from build123d import *

# Parameters (mm, degrees)
SKETCH_1_R             = 87
SM_BASE_FLANGE_1_DEPTH = 3
CUT_EXTRUDE_1_REACH    = 125.073
SKETCH_6_R             = 6.1
SKETCH_6_R_2           = 1
SKETCH_6_R_3           = 4.1
SKETCH_6_R_4           = 1.5
SKETCH_6_W             = 10
SKETCH_6_H             = 20
SKETCH_6_W_2           = 20
SKETCH_6_H_2           = 10
FILLET_1_R             = 3


# Sheet-metal steps are written as plain solids
with BuildPart() as part:
    # Sketch 1 → 基体-法兰1 (new body)
    with BuildSketch(Plane(origin=(0, 0, 0), x_dir=(1, 0, 0), z_dir=(0, 1, 0))):
        with Locations(Location((0, 0, 0), (0, 0, 270))):
            Circle(SKETCH_1_R)
    extrude(amount=-SM_BASE_FLANGE_1_DEPTH)

    # 草图6 → 切除-拉伸1 (cut, up to next)
    with BuildSketch(Plane(origin=(0, 0, 0), x_dir=(1, 0, 0), z_dir=(0, 1, 0)), mode=Mode.PRIVATE) as cut_extrude_1_sk1:
        with Locations(Location((0, 0, 0), (0, 0, 270))):
            Circle(SKETCH_6_R)
    cut_extrude_1_tool1 = extrude(cut_extrude_1_sk1.sketch, amount=-CUT_EXTRUDE_1_REACH, mode=Mode.PRIVATE) & part.part
    # 草图6 → 切除-拉伸1 (cut, up to next)
    with BuildSketch(Plane(origin=(0, 0, 0), x_dir=(1, 0, 0), z_dir=(0, 1, 0)), mode=Mode.PRIVATE) as cut_extrude_1_sk2:
        with Locations(Location((-8, 9.15, 0), (0, 0, 270))):
            Circle(SKETCH_6_R_2)
    cut_extrude_1_tool2 = extrude(cut_extrude_1_sk2.sketch, amount=-CUT_EXTRUDE_1_REACH, mode=Mode.PRIVATE) & part.part
    # 草图6 → 切除-拉伸1 (cut, up to next)
    with BuildSketch(Plane(origin=(0, 0, 0), x_dir=(1, 0, 0), z_dir=(0, 1, 0)), mode=Mode.PRIVATE) as cut_extrude_1_sk3:
        with Locations(Location((-7, 20.15, 0), (0, 0, 270))):
            Circle(SKETCH_6_R_2)
    cut_extrude_1_tool3 = extrude(cut_extrude_1_sk3.sketch, amount=-CUT_EXTRUDE_1_REACH, mode=Mode.PRIVATE) & part.part
    # 草图6 → 切除-拉伸1 (cut, up to next)
    with BuildSketch(Plane(origin=(0, 0, 0), x_dir=(1, 0, 0), z_dir=(0, 1, 0)), mode=Mode.PRIVATE) as cut_extrude_1_sk4:
        with Locations(Location((53.033008589, 53.033008589, 0), (0, 0, 270))):
            Circle(SKETCH_6_R_3)
    cut_extrude_1_tool4 = extrude(cut_extrude_1_sk4.sketch, amount=-CUT_EXTRUDE_1_REACH, mode=Mode.PRIVATE) & part.part
    # 草图6 → 切除-拉伸1 (cut, up to next)
    with BuildSketch(Plane(origin=(0, 0, 0), x_dir=(1, 0, 0), z_dir=(0, 1, 0)), mode=Mode.PRIVATE) as cut_extrude_1_sk5:
        with Locations(Location((-53.033008589, 53.033008589, 0), (0, 0, 270))):
            Circle(SKETCH_6_R_3)
    cut_extrude_1_tool5 = extrude(cut_extrude_1_sk5.sketch, amount=-CUT_EXTRUDE_1_REACH, mode=Mode.PRIVATE) & part.part
    # 草图6 → 切除-拉伸1 (cut, up to next)
    with BuildSketch(Plane(origin=(0, 0, 0), x_dir=(1, 0, 0), z_dir=(0, 1, 0)), mode=Mode.PRIVATE) as cut_extrude_1_sk6:
        with Locations(Location((53.033008589, -53.033008589, 0), (0, 0, 270))):
            Circle(SKETCH_6_R_3)
    cut_extrude_1_tool6 = extrude(cut_extrude_1_sk6.sketch, amount=-CUT_EXTRUDE_1_REACH, mode=Mode.PRIVATE) & part.part
    # 草图6 → 切除-拉伸1 (cut, up to next)
    with BuildSketch(Plane(origin=(0, 0, 0), x_dir=(1, 0, 0), z_dir=(0, 1, 0)), mode=Mode.PRIVATE) as cut_extrude_1_sk7:
        with Locations(Location((-53.033008589, -53.033008589, 0), (0, 0, 270))):
            Circle(SKETCH_6_R_3)
    cut_extrude_1_tool7 = extrude(cut_extrude_1_sk7.sketch, amount=-CUT_EXTRUDE_1_REACH, mode=Mode.PRIVATE) & part.part
    # 草图6 → 切除-拉伸1 (cut, up to next)
    with BuildSketch(Plane(origin=(0, 0, 0), x_dir=(1, 0, 0), z_dir=(0, 1, 0)), mode=Mode.PRIVATE) as cut_extrude_1_sk8:
        with Locations(Location((8, 9.15, 0), (0, 0, 270))):
            Circle(SKETCH_6_R_2)
    cut_extrude_1_tool8 = extrude(cut_extrude_1_sk8.sketch, amount=-CUT_EXTRUDE_1_REACH, mode=Mode.PRIVATE) & part.part
    # 草图6 → 切除-拉伸1 (cut, up to next)
    with BuildSketch(Plane(origin=(0, 0, 0), x_dir=(1, 0, 0), z_dir=(0, 1, 0)), mode=Mode.PRIVATE) as cut_extrude_1_sk9:
        with Locations(Location((7, 20.15, 0), (0, 0, 270))):
            Circle(SKETCH_6_R_2)
    cut_extrude_1_tool9 = extrude(cut_extrude_1_sk9.sketch, amount=-CUT_EXTRUDE_1_REACH, mode=Mode.PRIVATE) & part.part
    # 草图6 → 切除-拉伸1 (cut, up to next)
    with BuildSketch(Plane(origin=(0, 0, 0), x_dir=(1, 0, 0), z_dir=(0, 1, 0)), mode=Mode.PRIVATE) as cut_extrude_1_sk10:
        with Locations(Location((0, 27.15, 0), (0, 0, 270))):
            Circle(SKETCH_6_R_2)
    cut_extrude_1_tool10 = extrude(cut_extrude_1_sk10.sketch, amount=-CUT_EXTRUDE_1_REACH, mode=Mode.PRIVATE) & part.part
    # 草图6 → 切除-拉伸1 (cut, up to next)
    with BuildSketch(Plane(origin=(0, 0, 0), x_dir=(1, 0, 0), z_dir=(0, 1, 0)), mode=Mode.PRIVATE) as cut_extrude_1_sk11:
        with Locations(Location((-36.769552622, -36.769552622, 0), (0, 0, 270))):
            Circle(SKETCH_6_R_4)
    cut_extrude_1_tool11 = extrude(cut_extrude_1_sk11.sketch, amount=-CUT_EXTRUDE_1_REACH, mode=Mode.PRIVATE) & part.part
    # 草图6 → 切除-拉伸1 (cut, up to next)
    with BuildSketch(Plane(origin=(0, 0, 0), x_dir=(1, 0, 0), z_dir=(0, 1, 0)), mode=Mode.PRIVATE) as cut_extrude_1_sk12:
        with Locations(Location((-36.769552622, 36.769552622, 0), (0, 0, 270))):
            Circle(SKETCH_6_R_4)
    cut_extrude_1_tool12 = extrude(cut_extrude_1_sk12.sketch, amount=-CUT_EXTRUDE_1_REACH, mode=Mode.PRIVATE) & part.part
    # 草图6 → 切除-拉伸1 (cut, up to next)
    with BuildSketch(Plane(origin=(0, 0, 0), x_dir=(1, 0, 0), z_dir=(0, 1, 0)), mode=Mode.PRIVATE) as cut_extrude_1_sk13:
        with Locations(Location((36.769552622, 36.769552622, 0), (0, 0, 270))):
            Circle(SKETCH_6_R_4)
    cut_extrude_1_tool13 = extrude(cut_extrude_1_sk13.sketch, amount=-CUT_EXTRUDE_1_REACH, mode=Mode.PRIVATE) & part.part
    # 草图6 → 切除-拉伸1 (cut, up to next)
    with BuildSketch(Plane(origin=(0, 0, 0), x_dir=(1, 0, 0), z_dir=(0, 1, 0)), mode=Mode.PRIVATE) as cut_extrude_1_sk14:
        with Locations(Location((36.769552622, -36.769552622, 0), (0, 0, 270))):
            Circle(SKETCH_6_R_4)
    cut_extrude_1_tool14 = extrude(cut_extrude_1_sk14.sketch, amount=-CUT_EXTRUDE_1_REACH, mode=Mode.PRIVATE) & part.part
    # 草图6 → 切除-拉伸1 (cut, up to next)
    with BuildSketch(Plane(origin=(0, 0, 0), x_dir=(1, 0, 0), z_dir=(0, 1, 0)), mode=Mode.PRIVATE) as cut_extrude_1_sk15:
        with Locations((-35, 0)):
            Rectangle(SKETCH_6_W, SKETCH_6_H)
    cut_extrude_1_tool15 = extrude(cut_extrude_1_sk15.sketch, amount=-CUT_EXTRUDE_1_REACH, mode=Mode.PRIVATE) & part.part
    # 草图6 → 切除-拉伸1 (cut, up to next)
    with BuildSketch(Plane(origin=(0, 0, 0), x_dir=(1, 0, 0), z_dir=(0, 1, 0)), mode=Mode.PRIVATE) as cut_extrude_1_sk16:
        with Locations((35, 0)):
            Rectangle(SKETCH_6_W, SKETCH_6_H)
    cut_extrude_1_tool16 = extrude(cut_extrude_1_sk16.sketch, amount=-CUT_EXTRUDE_1_REACH, mode=Mode.PRIVATE) & part.part
    # 草图6 → 切除-拉伸1 (cut, up to next)
    with BuildSketch(Plane(origin=(0, 0, 0), x_dir=(1, 0, 0), z_dir=(0, 1, 0)), mode=Mode.PRIVATE) as cut_extrude_1_sk17:
        with Locations((0, -30)):
            Rectangle(SKETCH_6_W_2, SKETCH_6_H_2)
    cut_extrude_1_tool17 = extrude(cut_extrude_1_sk17.sketch, amount=-CUT_EXTRUDE_1_REACH, mode=Mode.PRIVATE) & part.part
    add(cut_extrude_1_tool1.solids().sort_by_distance((0, 0, 0))[0], mode=Mode.SUBTRACT)
    add(cut_extrude_1_tool2.solids().sort_by_distance((-8, 0, -9.15))[0], mode=Mode.SUBTRACT)
    add(cut_extrude_1_tool3.solids().sort_by_distance((-7, 0, -20.15))[0], mode=Mode.SUBTRACT)
    add(cut_extrude_1_tool4.solids().sort_by_distance((53.033009, 0, -53.033009))[0], mode=Mode.SUBTRACT)
    add(cut_extrude_1_tool5.solids().sort_by_distance((-53.033009, 0, -53.033009))[0], mode=Mode.SUBTRACT)
    add(cut_extrude_1_tool6.solids().sort_by_distance((53.033009, 0, 53.033009))[0], mode=Mode.SUBTRACT)
    add(cut_extrude_1_tool7.solids().sort_by_distance((-53.033009, 0, 53.033009))[0], mode=Mode.SUBTRACT)
    add(cut_extrude_1_tool8.solids().sort_by_distance((8, 0, -9.15))[0], mode=Mode.SUBTRACT)
    add(cut_extrude_1_tool9.solids().sort_by_distance((7, 0, -20.15))[0], mode=Mode.SUBTRACT)
    add(cut_extrude_1_tool10.solids().sort_by_distance((0, 0, -27.15))[0], mode=Mode.SUBTRACT)
    add(cut_extrude_1_tool11.solids().sort_by_distance((-36.769553, 0, 36.769553))[0], mode=Mode.SUBTRACT)
    add(cut_extrude_1_tool12.solids().sort_by_distance((-36.769553, 0, -36.769553))[0], mode=Mode.SUBTRACT)
    add(cut_extrude_1_tool13.solids().sort_by_distance((36.769553, 0, -36.769553))[0], mode=Mode.SUBTRACT)
    add(cut_extrude_1_tool14.solids().sort_by_distance((36.769553, 0, 36.769553))[0], mode=Mode.SUBTRACT)
    add(cut_extrude_1_tool15.solids().sort_by_distance((-35, 0, 0))[0], mode=Mode.SUBTRACT)
    add(cut_extrude_1_tool16.solids().sort_by_distance((35, 0, 0))[0], mode=Mode.SUBTRACT)
    add(cut_extrude_1_tool17.solids().sort_by_distance((0, 0, 30))[0], mode=Mode.SUBTRACT)

    # 圆角1
    fillet_1_edges = [part.edges().sort_by_distance(p)[0] for p in [
        (-10, -1.5, 35),
        (-10, -1.5, 25),
        (10, -1.5, 25),
        (10, -1.5, 35),
        (-30, -1.5, -10),
        (-30, -1.5, 10),
        (-40, -1.5, 10),
        (-40, -1.5, -10),
        (40, -1.5, -10),
        (40, -1.5, 10),
        (30, -1.5, 10),
        (30, -1.5, -10),
    ]]
    fillet(fillet_1_edges, radius=FILLET_1_R)


solid = part.part
Design review of the part built by this model. Coordinates are the model's own, in mm. Give positions to 0.01 mm unless a question says otherwise; leave off trailing zeros. Order: outer loops, then holes, each group sorted by start corner. A loop starts at its lowest first (then second) coordinate and runs counter-clockwise, first axis right, second up.
1. Add section B-B, the plane y = -1.95. State how many separate pieces and enclosed holes the cut face has, then the cut area to 3 significant figures.
Solution:
separate pieces: 1
enclosed holes: 17
area: 22,800 mm2
2. Add section A-A, the plane z = 0. State the section outline as (x, y) points, then the cut area to 3 significant figures.
Solution:
outline: (-87, -3) - (-40, -3) - (-40, 0) - (-87, 0) - close; (-30, -3) - (-6.1, -3) - (-6.1, 0) - (-30, 0) - close; (6.1, -3) - (30, -3) - (30, 0) - (6.1, 0) - close; (40, -3) - (87, -3) - (87, 0) - (40, 0) - close
area: 425 mm2
3. For pin 1 Ø0.9 at (x, y) = (-3, -2) entering from -Z; pin 2 Ø1.5 at (x, y) = (23, -0.5) entering from -Z; pin 3 Ø0.9 at (x, y) = (35, -2) entering from +Z, all flat-tipped, find the tip position at first contact; note any pin that passes through.
Solution:
pin 1: stops at z = -86.96
pin 2: stops at z = -84.11
pin 3: stops at z = 79.85
4. Add section D-D, the plane z = 46.5. State the section outline as (x, y) points.
Solution:
outline: (-73.53, -3) - (73.53, -3) - (73.53, 0) - (-73.53, 0) - close
5. Add section C-C, the plane x = 27.5. State the section outline as (y, z) points.
Solution:
outline: (-3, -82.54) - (0, -82.54) - (0, 82.54) - (-3, 82.54) - close
6. Mouldability with a two-part tool opening along Z and no side actions: class faces 1 (the cylindrical face through (57, -1, 52)), 2 (the cylindrical face through (86.26, -1.48, -11.33)), 3 (the flat face through (-18, 0, -1)) as +Z half, -Z half, draft (parallel to the pull), parting line (faces both ways), or undercut.
Solution:
face 1: undercut
face 2: parting line
face 3: draft
7. To check wall thickness, follow L1, parallel to Z at x = 52.5, y = -2; L2, parallel to Z at x = -53, y = -1.05; L3, parallel to X at y = -1.8, z = -20.15. State the ranges of each line that lie inside material, in increasing order.
Solution:
L1: z = -69.37 to -57.1, -48.97 to 48.97, 57.1 to 69.37
L2: z = -68.99 to -57.13, -48.93 to 48.93, 57.13 to 68.99
L3: x = -84.63 to -8, -6 to 6, 8 to 84.63
